from build123d import *

# Parameters (mm, degrees)
SKETCH1_W           = 195.2625
SKETCH1_H           = 33.3375
SKETCH1_R           = 3.175
BOSS_EXTRUDE1_DEPTH = 17.78
SKETCH2_R           = 3.96875
CUT_EXTRUDE1_DEPTH  = 33.3375
SKETCH3_R           = 4.7625
CUT_EXTRUDE2_DEPTH  = 4.7752
CUT_EXTRUDE3_DEPTH  = 17.78


with BuildPart() as part:
    # Sketch1 → Boss-Extrude1 (new body)
    with BuildSketch(Plane.XY):
        with Locations((-88.9, 0)):
            Rectangle(SKETCH1_W, SKETCH1_H)
        Circle(SKETCH1_R, mode=Mode.SUBTRACT)
        with Locations((-177.8, 0)):
            Circle(SKETCH1_R, mode=Mode.SUBTRACT)
        with Locations((-88.9, 0)):
            Circle(SKETCH1_R, mode=Mode.SUBTRACT)
    extrude(amount=-BOSS_EXTRUDE1_DEPTH)

    # Sketch2 → Cut-Extrude1 (cut)
    with BuildSketch(Plane(origin=(0, 16.66875, 0), x_dir=(1, 0, 0), z_dir=(0, 1, 0))):
        with Locations(Location((-12.7, 8.89, 0), (0, 0, 270))):
            Circle(SKETCH2_R)
        with Locations(Location((-63.5, 8.89, 0), (0, 0, 270))):
            Circle(SKETCH2_R)
        with Locations(Location((-114.3, 8.89, 0), (0, 0, 270))):
            Circle(SKETCH2_R)
        with Locations(Location((-165.1, 8.89, 0), (0, 0, 270))):
            Circle(SKETCH2_R)
    extrude(amount=-CUT_EXTRUDE1_DEPTH, mode=Mode.SUBTRACT)

    # Sketch3 → Cut-Extrude2 (cut)
    with BuildSketch(Plane.XY):
        Circle(SKETCH3_R)
        with Locations((-88.9, 0)):
            Circle(SKETCH3_R)
        with Locations((-177.8, 0)):
            Circle(SKETCH3_R)
    extrude(amount=-CUT_EXTRUDE2_DEPTH, mode=Mode.SUBTRACT)

    # Sketch5 → Cut-Extrude3 (cut)
    with BuildSketch(Plane.XY):
        with BuildLine():
            Line((0, -16.66875), (8.73125, -16.66875))
            Line((8.73125, -16.66875), (8.73125, 16.66875))
            Line((8.73125, 16.66875), (0, 16.66875))
            Line((0, 16.66875), (0, 10.622546022))
            ThreePointArc((0, 10.622546022), (0.546012526, 9.049137635), (1.949302326, 8.152186482))
            ThreePointArc((1.949302326, 8.152186482), (8.382, 0), (1.949302326, -8.152186482))
            ThreePointArc((1.949302326, -8.152186482), (0.546012526, -9.049137635), (0, -10.622546022))
            Line((0, -10.622546022), (0, -16.66875))
        make_face()
        with BuildLine():
            Line((-22.86, -12.7), (-53.34, -12.7))
            ThreePointArc((-53.34, -12.7), (-55.136051224, -11.956051224), (-55.88, -10.16))
            Line((-55.88, -10.16), (-55.88, 10.16))
            ThreePointArc((-55.88, 10.16), (-55.136051224, 11.956051224), (-53.34, 12.7))
            Line((-53.34, 12.7), (-22.86, 12.7))
            ThreePointArc((-22.86, 12.7), (-21.063948776, 11.956051224), (-20.32, 10.16))
            Line((-20.32, 10.16), (-20.32, -10.16))
            ThreePointArc((-20.32, -10.16), (-21.063948776, -11.956051224), (-22.86, -12.7))
        make_face()
        with BuildLine():
            Line((-85.011936327, -9.38661605), (-85.011936327, -12.7))
            Line((-85.011936327, -12.7), (-76.883936327, -12.7))
            ThreePointArc((-76.883936327, -12.7), (-75.087885103, -11.956051224), (-74.343936327, -10.16))
            Line((-74.343936327, -10.16), (-74.343936327, 10.16))
            ThreePointArc((-74.343936327, 10.16), (-75.087885103, 11.956051224), (-76.883936327, 12.7))
            Line((-76.883936327, 12.7), (-85.011936327, 12.7))
            Line((-85.011936327, 12.7), (-85.011936327, 9.38661605))
            ThreePointArc((-85.011936327, 9.38661605), (-78.74, 0), (-85.011936327, -9.38661605))
        make_face()
        with BuildLine():
            Line((-100.916063673, 12.7), (-92.788063673, 12.7))
            Line((-92.788063673, 12.7), (-92.788063673, 9.38661605))
            ThreePointArc((-92.788063673, 9.38661605), (-99.06, 0), (-92.788063673, -9.38661605))
            Line((-92.788063673, -9.38661605), (-92.788063673, -12.7))
            Line((-92.788063673, -12.7), (-100.916063673, -12.7))
            ThreePointArc((-100.916063673, -12.7), (-102.712114897, -11.956051224), (-103.456063673, -10.16))
            Line((-103.456063673, -10.16), (-103.456063673, 10.16))
            ThreePointArc((-103.456063673, 10.16), (-102.712114897, 11.956051224), (-100.916063673, 12.7))
        make_face()
        with BuildLine():
            Line((-154.94, 12.7), (-124.46, 12.7))
            ThreePointArc((-124.46, 12.7), (-122.663948776, 11.956051224), (-121.92, 10.16))
            Line((-121.92, 10.16), (-121.92, -10.16))
            ThreePointArc((-121.92, -10.16), (-122.663948776, -11.956051224), (-124.46, -12.7))
            Line((-124.46, -12.7), (-154.94, -12.7))
            ThreePointArc((-154.94, -12.7), (-156.736051224, -11.956051224), (-157.48, -10.16))
            Line((-157.48, -10.16), (-157.48, 10.16))
            ThreePointArc((-157.48, 10.16), (-156.736051224, 11.956051224), (-154.94, 12.7))
        make_face()
        with BuildLine():
            Line((-186.53125, -16.66875), (-186.53125, 16.66875))
            Line((-186.53125, 16.66875), (-177.8, 16.66875))
            Line((-177.8, 16.66875), (-177.8, 10.622546022))
            ThreePointArc((-177.8, 10.622546022), (-178.346012526, 9.049137635), (-179.749302326, 8.152186482))
            ThreePointArc((-179.749302326, 8.152186482), (-186.182, 0), (-179.749302326, -8.152186482))
            ThreePointArc((-179.749302326, -8.152186482), (-178.346012526, -9.049137635), (-177.8, -10.622546022))
            Line((-177.8, -10.622546022), (-177.8, -16.66875))
            Line((-177.8, -16.66875), (-186.53125, -16.66875))
        make_face()
    extrude(amount=-CUT_EXTRUDE3_DEPTH, mode=Mode.SUBTRACT)


solid = part.part
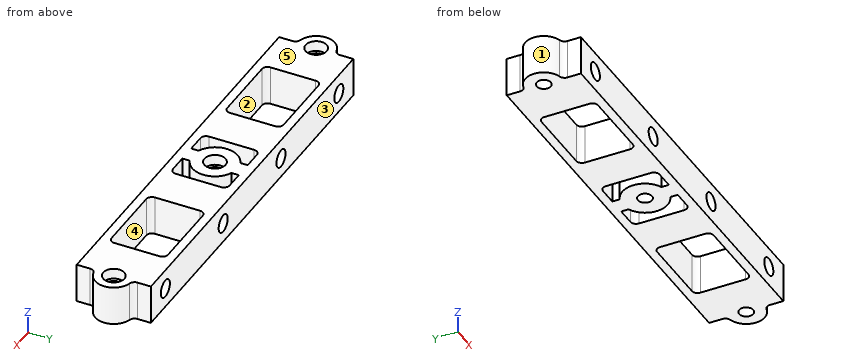
Verification items for the finished model (mm, model axes). Face numbers are marked on the shaded views. A direction names the side the tool comes from. Round coordinates to 2 decimals unless told otherwise and drop trailing zeros. Loops run counter-clockwise (first coordinate to the right, second up) from the corner with the lowest first, then second, coordinate; pieces in that order, holes last. Notation, with made-up numbers: (46.5, -6) - (57.5, -6) arc R36 cw to (57.5, 30) - close; hole circle Ø3 at (60.5, 17). An arc over 180 degrees is marked (long way). Use a Markdown table: item, result. Add a question column.
1. Thickness scan on probe 1 along X at (y, z) = (15, -6); probe 2 along Y at (x, z) = (-39, -9.5); probe 3 along Y at (x, z) = (-80.5, -9.75). Record the ranges inside material, lowest first. Write a range as [from, to].
2. Access from +Z, -Z, +X, -X, +Y, -Y to the whole of each face (thin tool, end or side, straight path). Record for the marked faces 4 and 5.
3. Section check C-C, the plane z = -9.5. Give the number of separate pieces and of enclosed holes in the cut face, plus the area to 3 significant figures.
4. Release check for a two-part mould opening along X. For the marked faces 1, 2 and 3 record: released by +X, released by -X, zero draft, split by the parting line, or undercut.
5. Section check B-B, the plane x = -88.9. Record the boundary of the cut face in (y, z) (1 decimal).
6. Section check A-A, the plane x = -12.7. Record the boundary of the cut face in (y, z), plus the area to 3 significant figures.
7. Gauge pin test, flat ends, axial feed: pin 1 (6 mm diameter, centred on y = 10, z = -15, fed in from +X); pin 2 (7.5 mm diameter, centred on x = -87, y = 1.5, fed in from +Z); pin 3 (3 mm diameter, centred on y = 4, z = -3.5, fed in from +X); pin 4 (5 mm diameter, centred on x = -88.9, y = 0, fed in from +Z). Record the tip position at first contact, or that the pin passes through.
Checks:
| question | item | result |
|---|---|---|
| 1 | probe 1 | x = [-177.8, -167.82], [-162.38, -117.02], [-111.58, -66.22], [-60.78, -15.42], [-9.98, 0] |
| 1 | probe 2 | y = [-16.67, -12.7], [12.7, 16.67] |
| 1 | probe 3 | y = [-16.67, -12.7], [-5.72, 5.72], [12.7, 16.67] |
| 2 | face 4 | +Z, -Z |
| 2 | face 5 | +Z, +X, -X, +Y, -Y |
| 3 | separate pieces | 5 |
| 3 | enclosed holes | 7 |
| 3 | area | 2,850 mm^2 |
| 4 | face 1 | released by -X |
| 4 | face 2 | undercut |
| 4 | face 3 | zero draft |
| 5 | outline | (-16.7, -17.8) - (-3.2, -17.8) - (-3.2, -4.8) - (-4.8, -4.8) - (-4.8, 0) - (-16.7, 0) - close; (3.2, -17.8) - (16.7, -17.8) - (16.7, 0) - (4.8, 0) - (4.8, -4.8) - (3.2, -4.8) - close |
| 6 | outline | (-16.67, -17.78) - (16.67, -17.78) - (16.67, -12.86) - (-16.67, -12.86) - close; (-16.67, -4.92) - (16.67, -4.92) - (16.67, 0) - (-16.67, 0) - close |
| 6 | area | 328 mm^2 |
| 7 | pin 1 | stops at x = 4.61 |
| 7 | pin 2 | stops at z = 0 |
| 7 | pin 3 | stops at x = 8 |
| 7 | pin 4 | passes through |
